Source: CAD feature listing. Evaluate the final solid. Frame: model axes, mm. A direction names the side the tool comes from. Give positions to 0.01 mm unless a question says otherwise; leave off trailing zeros. Order: outer loops, then holes, each group sorted by start corner. A loop starts at its lowest first (then second) coordinate and runs counter-clockwise, first axis right, second up. Notation, with made-up numbers: (64, 45.25) -> (74, 45.25) arc R13 cw to (74, 56.25) -> close; hole circle Ø1 at (-23.5, 12). An arc over 180 degrees is marked (long way). Answer in a Markdown table with one row per item.
```python
from build123d import *

# Parameters (mm, degrees)
F0_R     = 3.8
F1_DEPTH = 8.9
F2_R     = 10
F3_DEPTH = 2
F4_R     = 2.5
F5_DEPTH = 8.3
F6_R     = 5.65
F7_DEPTH = 1.4


with BuildPart() as f1:
    # F0 (on Top) → F1 (new body)
    with BuildSketch(Plane.XY):
        Circle(F0_R)
    extrude(amount=F1_DEPTH)

    # F2 (on face) → F3 (join)
    with BuildSketch(Plane.XY.offset(8.9)):
        Circle(F2_R)
    extrude(amount=F3_DEPTH)

    # F4 (on face) → F5 (cut)
    with BuildSketch(Plane(origin=(0, 0, 0), x_dir=(1, 0, 0), z_dir=(0, 0, -1))):
        Circle(F4_R)
    extrude(amount=-F5_DEPTH, mode=Mode.SUBTRACT)

    # F6 (on face) → F7 (join)
    with BuildSketch(Plane(origin=(0, 0, 8.9), x_dir=(1, 0, 0), z_dir=(0, 0, -1))):
        Circle(F6_R)
    extrude(amount=F7_DEPTH)


solid = f1.part
```
(1) Section query C-C (z = 2.25). Return the cut outline in (x, y).
A:
| item | result |
|---|---|
| outline | circle Ø7.6 at (0, 0); hole circle Ø5 at (0, 0) |
(2) Section query A-A (x = 0). Return the cut outline in (y, z), plus the area to 3 significant figures.
A:
| item | result |
|---|---|
| outline | (-10, 8.9) -> (-5.65, 8.9) -> (-5.65, 7.5) -> (-3.8, 7.5) -> (-3.8, 0) -> (-2.5, 0) -> (-2.5, 7.5) -> (2.5, 7.5) -> (2.5, 0) -> (3.8, 0) -> (3.8, 7.5) -> (5.65, 7.5) -> (5.65, 8.9) -> (10, 8.9) -> (10, 10.9) -> (-10, 10.9) -> close |
| area | 75.3 mm^2 |
(3) Pull-direction query (X, two-part tool) for faces 1 (the flat face through (0, 0, 7.5)), 2 (the flat face through (0, 0, 10.9)), 3 (the cylindrical face through (-0.54, 2.44, 3.7)), 4 (the cylindrical face through (5.39, -1.7, 8.21)); classes: +X half, -X half, draft (parallel to the pull), parting line (faces both ways), or undercut.
A:
| item | result |
|---|---|
| face 1 | undercut |
| face 2 | draft |
| face 3 | undercut |
| face 4 | parting line |
(4) Ray query, probe 1 along X at (y, z) = (0, 2.75); probe 2 along Z at (x, y) = (3.5, -5). Return the intervals inside material, ascending.
A:
| item | result |
|---|---|
| probe 1 | x = -3.8 to -2.5, 2.5 to 3.8 |
| probe 2 | z = 8.9 to 10.9 |
(5) First-contact query: pin 1 Ø5 at (x, y) = (1.5, -2.5) entering from -Z; pin 2 Ø3 at (y, z) = (-2, 1.5) entering from -X; pin 3 Ø1.5 at (x, z) = (-6, 6) entering from -Y; pin 4 Ø2 at (y, z) = (-2, 3) entering from -X. Flat tips, straight axial feed; report the tip coordinate or a pass-through.
A:
| item | result |
|---|---|
| pin 1 | stops at z = 0 |
| pin 2 | stops at x = -3.77 |
| pin 3 | passes through |
| pin 4 | stops at x = -3.67 |
(6) Section query D-D (z = 8.25). Return the cut outline in (x, y).
A:
| item | result |
|---|---|
| outline | circle Ø11.3 at (0, 0) |
(7) Access query for faces 5 (the flat face through (4, 1, 7.5)), 6 (the flat face through (-0.9, -2.5, 0)). Directions: +Z, -Z, +X, -X, +Y, -Y. A direction counts if a zero-diameter tool reaches every point of the face in a straight line with its end or side. Return the directions, or none.
A:
| item | result |
|---|---|
| face 5 | -Z |
| face 6 | -Z, +X, -X, +Y, -Y |
